```python
from build123d import *

# Parameters (mm, degrees)
F2_DEPTH  = 20
F3_DEPTH  = 25
F6_DEPTH  = 25
F9_DEPTH  = 25
F12_DEPTH = 20
F15_DEPTH = 20
F18_DEPTH = 20


with BuildPart() as f2:
    # F0 (on Top) → F2 (new body)
    with BuildSketch(Plane.XY):
        Polygon((72.1636915906, -40.0095078308), (-1.4325956209, 82.5003440637), (-70.7310959697, -42.4908362329), align=None)
    extrude(amount=-F2_DEPTH)

    # F1 (on face) → F3 (join)
    with BuildSketch(Plane.XY):
        Polygon((63.7132421591, -36.7848575115), (0, 73.569715023), (-7.9415651396, 59.8145207096), (39.8885467402, -23.0296631981), (-55.7716770195, -23.0296631981), (-63.7132421591, -36.7848575115), align=None)
    extrude(amount=F3_DEPTH)

    # F5 (on offset) → F6 (join)
    with BuildSketch(Plane.XY.offset(25)):
        Polygon((-63.5274310143, -36.5936169448), (63.4547173977, -36.7195606232), (55.453214499, -22.828752175), (40.0054380298, -22.828752175), (-39.7729983351, -23.2313495358), (-0.2324396947, 46.0601017108), (7.7318175716, 60.0167822194), (0.0727136166, 73.3131775679), align=None)
    extrude(amount=F6_DEPTH)

    # F8 (on offset) → F9 (join)
    with BuildSketch(Plane.XY.offset(50)):
        Polygon((0.0727136166, 73.3131775679), (-63.5274310143, -36.5936169448), (-47.9317654972, -36.6090850677), (0, 46.2213350785), (48.4369544614, -36.7046656767), (63.4547173977, -36.7195606232), align=None)
    extrude(amount=F9_DEPTH)

    # F11 (on offset) → F12 (join)
    with BuildSketch(Plane(origin=(-0.0363568083, -36.656588784, 0), x_dir=(0.9999995081, -0.0009918214, 0), z_dir=(-0.0009918214, -0.9999995081, 0))):
        Polygon((-31.1529804021, 43.7380857766), (-48.2164211571, 9.2830741778), (45.9606572986, 9.2830741778), (45.9606572986, 14.7767344154), (-36.6358867937, 14.7767344154), (-22.2931168973, 43.7380857766), align=None)
    extrude(amount=F12_DEPTH)

    # F14 (on offset) → F15 (join)
    with BuildSketch(Plane(origin=(-31.7273586988, 18.3597803116, 0), x_dir=(-0.5008586966, -0.8655290671, 0), z_dir=(-0.8655290671, 0.5008586966, 0))):
        Polygon((-51.3164810836, 24.628393352), (-49.2495509186, 24.628393352), (-43.5906848585, 24.628393352), (50.7504490814, 24.628393352), (50.7504490814, 29.7592282616), (-49.2495509186, 29.7592282616), (-56.9396201191, 49.6568456292), (-60.9895251691, 49.6568456292), align=None)
    extrude(amount=F15_DEPTH)

    # F17 (on offset) → F18 (join)
    with BuildSketch(Plane(origin=(31.8566210796, 18.3924287558, 0), x_dir=(-0.5, 0.8660254038, 0), z_dir=(0.8660254038, 0.5, 0))):
        Polygon((-31.7721163192, 72.7189217287), (-42.6499355114, 72.7189217287), (-58.2169406468, 3.7218167854), (53.5177626068, 3.7218167854), (-2.5316273462, 72.3955608765), (-15.0649024936, 72.3955608765), (34.463509317, 11.7115555596), (-45.536490683, 11.7115555596), align=None)
    extrude(amount=F18_DEPTH)


solid = f2.part
```
The listing builds one solid part. Answer for the finished solid, in the listing's coordinates (mm). A direction names the side the tool comes from. Give positions to 0.01 mm unless a question says otherwise; leave off trailing zeros. Order: outer loops, then holes, each group sorted by start corner. A loop starts at its lowest first (then second) coordinate and runs counter-clockwise, first axis right, second up.
1) Find section C-C on x = -16.5. Write down the section's boundary in (y, z), then the cut area to 3 significant figures.
Reported:
outline: (-56.64, 9.28) - (-36.78, 9.28) - (-36.78, 0) - (-41.55, 0) - (-41.55, -20) - (55.32, -20) - (55.32, 0) - (-23.03, 0) - (-23.03, 25) - (-23.11, 25) - (-23.11, 50) - (-36.64, 50) - (-36.64, 25) - (-36.78, 25) - (-36.78, 14.78) - (-56.64, 14.78) - close; (17.55, 25) - (44.67, 25) - (44.67, 24.63) - (68.84, 24.63) - (80.01, 49.66) - (75.33, 49.66) - (66.45, 29.76) - (44.67, 29.76) - (44.67, 75) - (17.71, 75) - (17.71, 50) - (17.55, 50) - close
area: 4,300 mm2
2) For faces 1 (the face through (59, -9, 72.719)), 2 (the face through (27, 16, 50)), 3 (the face through (27.453, 45.74, 37.578)), determine the directions among +Z, -Z, +X, -X, +Y, -Y from which every point of the face is accessible in a straight line to the end or side of a thin tool.
Reported:
face 1: +Z, +X, +Y
face 2: none
face 3: +Z, +Y
3) Consider line 1 along Z through (x, y) = (44, -7); line 2 along Y through (x, z) = (-14, 47); line 3 along Z through (x, y) = (-34, 0). Determine where each line is inside the solid, lowest interval first.
Reported:
line 1: z = -20 to 25, 50 to 75
line 2: y = -36.64 to -23.1, 21.93 to 48.99, 72.7 to 77.38
line 3: z = -20 to 0, 25 to 75
4) Determine the mould class of faces 4 (the face through (-35.597, 20.88, -9.86)), 5 (the face through (-31.424, 18.883, 24.817)), 6 (the face through (0, 7, -20)), 7 (the face through (35.72, 31.42, 42.48)) for opening direction Y: pulls with the +Y half, pulls with the -Y half, needs draft (parallel to the pull), parting line crosses it, or undercut.
Reported:
face 4: pulls with the +Y half
face 5: undercut
face 6: needs draft
face 7: undercut
5) Given P1, Ø5, axis at y = -20, z = 19, coming from the -X side; P2, Ø1, axis at x = 4.5, z = 55, coming from the -Y side; P3, Ø16, axis at x = -12.5, y = -48, coming from the +Z side, each flat-ended and moving along its own axis, determine where each tip first touches the part or whether it passes through.
Reported:
P1: stops at x = 36.7
P2: stops at y = 37.66
P3: stops at z = 14.78
6) Find section B-B on z = 64. Write down the section's boundary in (x, y), then the cut area to 3 significant figures.
Reported:
outline: (-63.53, -36.59) - (-47.93, -36.61) - (0, 46.22) - (48.44, -36.7) - (63.45, -36.72) - (0.07, 73.31) - close; (29.7, 22.13) - (35.96, 11.28) - (53.28, 21.28) - (47.02, 32.13) - close; (48.73, -10.83) - (54.17, -20.25) - (71.49, -10.25) - (66.05, -0.83) - close
area: 3,460 mm2
7) Find section A-A on y = 10. Give the number of separate pieces and of enclosed holes in the cut face, then the cut area to 3 significant figures.
Reported:
separate pieces: 4
enclosed holes: 0
area: 3,580 mm2
